Input: part model. Units: mm. Frame: model coordinates. A direction names the side the tool comes from. Round coordinates to 2 decimals unless told otherwise and drop trailing zeros. Write each loop counter-clockwise with the first axis right and the second up, starting at its lowest first coordinate (ties: lowest second). Pieces come first, ordered by that corner, then holes. Notation, with made-up numbers: (62, 42.25) -> (72, 42.25) arc R10 ccw to (72, 46.25) -> close; hole circle Ø6 at (71.25, 87.25). An arc over 180 degrees is marked (long way). Use CSV: the item, a comma, the result in double quotes.
```python
from build123d import *

# Parameters (mm, degrees)
SKETCH1_W           = 20
SKETCH1_H           = 10
SKETCH1_W_2         = 10
SKETCH1_H_2         = 13.195504549
SKETCH1_H_3         = 13.608990902
SKETCH1_H_4         = 113.195504549
BOSS_EXTRUDE1_DEPTH = 5
SKETCH1_3_W         = 20
SKETCH1_3_H         = 10
SKETCH1_3_W_2       = 10
SKETCH1_3_H_2       = 13.608990902
BOSS_EXTRUDE2_DEPTH = 20
SKETCH1_5_W         = 10
SKETCH1_5_H         = 113.195504549
BOSS_EXTRUDE3_DEPTH = 10
SKETCH3_R           = 4
CUT_EXTRUDE1_DEPTH  = 10
FILLET1_R           = 10
FILLET2_R           = 5
FILLET3_R           = 7
FILLET4_R           = 7
FILLET5_R           = 7


# Some blends are built 0.0001 mm under size
with BuildPart() as part:
    # Sketch1 → Boss-Extrude1 (new body)
    with BuildSketch(Plane(origin=(0, 0, 0), x_dir=(1, 0, 0), z_dir=(0, 1, 0))):
        Polygon((60, -8.515763432), (44.667493795, -8.515763432), (40, -8.515763432), (40, -18.515763432), (60, -18.515763432), align=None)
        Polygon((40, -8.515763432), (44.667493795, -8.515763432), (60, -8.515763432), (60, 1.484236568), (5, 1.484236568), (-5, 1.484236568), (-60, 1.484236568), (-60, -8.515763432), (-40, -8.515763432), align=None)
        with Locations((-50, -13.515763432)):
            Rectangle(SKETCH1_W, SKETCH1_H)
        with Locations((0, 8.081988842)):
            Rectangle(SKETCH1_W_2, SKETCH1_H_2)
        with Locations((0, 21.484236568)):
            Rectangle(SKETCH1_W_2, SKETCH1_H_3)
        with Locations((0, 84.886484294)):
            Rectangle(SKETCH1_W_2, SKETCH1_H_4)
    extrude(amount=BOSS_EXTRUDE1_DEPTH)

    # Sketch1<3> → Boss-Extrude2 (add)
    with BuildSketch(Plane(origin=(0, 0, 0), x_dir=(1, 0, 0), z_dir=(0, 1, 0))):
        with Locations((-50, -13.515763432)):
            Rectangle(SKETCH1_3_W, SKETCH1_3_H)
        Polygon((60, -8.515763432), (44.667493795, -8.515763432), (40, -8.515763432), (40, -18.515763432), (60, -18.515763432), align=None)
        with Locations((0, 21.484236568)):
            Rectangle(SKETCH1_3_W_2, SKETCH1_3_H_2)
    extrude(amount=BOSS_EXTRUDE2_DEPTH)

    # Sketch1<5> → Boss-Extrude3 (add)
    with BuildSketch(Plane(origin=(0, 0, 0), x_dir=(1, 0, 0), z_dir=(0, 1, 0))):
        with Locations((0, 84.886484294)):
            Rectangle(SKETCH1_5_W, SKETCH1_5_H)
    extrude(amount=BOSS_EXTRUDE3_DEPTH)

    # Sketch3 → Cut-Extrude1 (cut)
    with BuildSketch(Plane(origin=(5, 0, 0), x_dir=(0, 0, -1), z_dir=(1, 0, 0))):
        with Locations((21.484236568, 13)):
            Circle(SKETCH3_R)
        with BuildLine():
            Line((120.663634314, 6.570050981), (119.289130035, 10))
            Line((119.289130035, 10), (125.484236568, 10))
            Line((125.484236568, 10), (125.484236568, 7.5))
            ThreePointArc((125.484236568, 7.5), (123.457784012, 5.045259114), (120.663634314, 6.570050981))
        make_face()
        with BuildLine():
            Line((133.984236568, 7.5), (133.984236568, 10))
            Line((133.984236568, 10), (127.789130035, 10))
            Line((127.789130035, 10), (129.163634314, 6.570050981))
            ThreePointArc((129.163634314, 6.570050981), (131.957784012, 5.045259114), (133.984236568, 7.5))
        make_face()
        Polygon((141.484236568, 6), (139.984236568, 4.5), (141.484236568, 3), align=None)
        with BuildLine():
            Line((112.163634314, 6.570050981), (110.789130035, 10))
            Line((110.789130035, 10), (116.984236568, 10))
            Line((116.984236568, 10), (116.984236568, 7.5))
            ThreePointArc((116.984236568, 7.5), (114.957784012, 5.045259114), (112.163634314, 6.570050981))
        make_face()
        with BuildLine():
            Line((103.663634314, 6.570050981), (102.289130035, 10))
            Line((102.289130035, 10), (108.484236568, 10))
            Line((108.484236568, 10), (108.484236568, 7.5))
            ThreePointArc((108.484236568, 7.5), (106.457784012, 5.045259114), (103.663634314, 6.570050981))
        make_face()
        with BuildLine():
            Line((95.163634314, 6.570050981), (93.789130035, 10))
            Line((93.789130035, 10), (99.984236568, 10))
            Line((99.984236568, 10), (99.984236568, 7.5))
            ThreePointArc((99.984236568, 7.5), (97.957784012, 5.045259114), (95.163634314, 6.570050981))
        make_face()
        with BuildLine():
            Line((86.663634314, 6.570050981), (85.289130035, 10))
            Line((85.289130035, 10), (91.484236568, 10))
            Line((91.484236568, 10), (91.484236568, 7.5))
            ThreePointArc((91.484236568, 7.5), (89.457784012, 5.045259114), (86.663634314, 6.570050981))
        make_face()
    extrude(amount=-CUT_EXTRUDE1_DEPTH, mode=Mode.SUBTRACT)

    # Fillet1
    fillet1_edges = [part.edges().sort_by_distance(p)[0] for p in [
        (0, 5, -14.679741117),
    ]]
    fillet(fillet1_edges, radius=FILLET1_R)

    # Fillet2
    fillet2_edges = [part.edges().sort_by_distance(p)[0] for p in [
        (-50, 20, 8.515763432),
        (-50, 20, 18.515763432),
        (50, 20, 8.515763432),
        (50, 20, 18.515763432),
    ]]
    fillet(fillet2_edges, radius=FILLET2_R - 0.0001)  # a hair under: the kernel refuses the full size

    # Fillet3
    fillet3_edges = [part.edges().sort_by_distance(p)[0] for p in [
        (0, 20, -14.679741117),
    ]]
    fillet(fillet3_edges, radius=FILLET3_R)

    # Fillet4
    # the kernel refuses this fillet: 7 mm, written as the material it takes off along each edge
    with BuildSketch(Plane(origin=(22.486690858, 20, -28.288732019), x_dir=(0, 0, 1), z_dir=(-1, 0, 0))) as fillet4_piece_1:
        with BuildLine():
            CenterArc((7, -6.994676343), FILLET4_R, 92.234709992, 87.765290008)
            Line((0, -6.994676343), (-0.14, -6.994676343))
            Line((-0.14, -6.994676343), (-0.14, 0))
            Line((-0.14, 0), (0, 0.14))
            ThreePointArc((0, 0.14), (3.363523943, 0.14), (6.721588844, 0.139893527))
            Line((6.721588844, 0.139893527), (6.727047886, 0))
        make_face()
    extrude(amount=44.973381715, mode=Mode.SUBTRACT)

    # Fillet5
    fillet5_edges = [part.edges().sort_by_distance(p)[0] for p in [
        (-60, 2.5, -1.484236568),
        (60, 2.5, -1.484236568),
    ]]
    fillet(fillet5_edges, radius=FILLET5_R)


solid = part.part
```
Item 1: Section query C-C on x = 11. Return the cut outline in (y, z), plus the area to 3 significant figures.
Worked answers:
outline,"(0, -1.48) -> (5, -1.48) -> (5, 8.52) -> (0, 8.52) -> close"
area,"50.0 mm²"
Item 2: Set-up query: faces 1 (the face through (29, 2, -1.484)), 2 (the face through (0.07, 8.261, -102.986)), 3 (the face through (-1, 2, 8.516)). Return all of +Z, -Z, +X, -X, +Y, -Y with unobstructed straight access to the full face (end or side cutting, diameter ignored); none if empty.
Worked answers:
face 1,"-Z, +X, +Y, -Y"
face 2,"+X, -X, +Y"
face 3,"+Z, +Y, -Y"
Item 3: Line query: line 1 (Z direction, x = 42, y = 11.25); line 2 (X direction, y = 6.5, z = -62); line 3 (Y direction, x = -6, z = 5.5). Output: solid intervals per line, ascending.
Worked answers:
line 1,"z = 8.52 to 18.52"
line 2,"x = -5 to 5"
line 3,"y = 0 to 5"
Item 4: First-contact query: pin 1 Ø6 at (y, z) = (6.5, -56.5) entering from +X; pin 2 Ø8 at (x, y) = (40.5, 7.5) entering from -Z; pin 3 Ø1.2 at (x, y) = (-0.5, 8.5) entering from +Z. Flat tips, straight axial feed; report the tip coordinate or a pass-through.
Worked answers:
pin 1,"stops at x = 5"
pin 2,"stops at z = -1.48"
pin 3,"stops at z = -11.72"
Item 5: Pull-direction query (Z, two-part tool) for faces 4 (the face through (0, 10, -57)), 5 (the face through (0, 8, -141.484)), 6 (the face through (0.07, 8.261, -119.986)); classes: +Z half, -Z half, draft (parallel to the pull), parting line (faces both ways), or undercut.
Worked answers:
face 4,"draft"
face 5,"-Z half"
face 6,"undercut"
Item 6: Section query B-B on z = -62.5. Return the cut outline in (x, y), plus the area to 3 significant figures.
Worked answers:
outline,"(-5, 0) -> (5, 0) -> (5, 10) -> (-5, 10) -> close"
area,"100 mm²"
